```python
from build123d import *

# Parameters (mm, degrees)
SALIENTE_EXTRUIR1_DEPTH = 200


with BuildPart() as part:
    # Croquis1 → Saliente-Extruir1 (new, symmetric)
    with BuildSketch(Plane.XY):
        with BuildLine():
            Line((-10, 8.5), (-10, 2.3))
            Line((-10, 2.3), (-8.2, 2.3))
            Line((-8.2, 2.3), (-8.2, 5.5))
            Line((-8.2, 5.5), (-6.348528137, 5.5))
            Line((-6.348528137, 5.5), (-4.485786438, 3.6372583))
            ThreePointArc((-4.485786438, 3.6372583), (-4.052240935, 2.988411603), (-3.9, 2.223044738))
            Line((-3.9, 2.223044738), (-3.9, 0))
            Line((-3.9, 0), (-3.9, -2.223044738))
            ThreePointArc((-3.9, -2.223044738), (-4.052240935, -2.988411603), (-4.485786438, -3.6372583))
            Line((-4.485786438, -3.6372583), (-6.348528137, -5.5))
            Line((-6.348528137, -5.5), (-8.2, -5.5))
            Line((-8.2, -5.5), (-8.2, -2.3))
            Line((-8.2, -2.3), (-10, -2.3))
            Line((-10, -2.3), (-10, -8.5))
            ThreePointArc((-10, -8.5), (-9.560660172, -9.560660172), (-8.5, -10))
            Line((-8.5, -10), (-2.3, -10))
            Line((-2.3, -10), (-2.3, -8.2))
            Line((-2.3, -8.2), (-5.5, -8.2))
            Line((-5.5, -8.2), (-5.5, -6.348528137))
            Line((-5.5, -6.348528137), (-3.6372583, -4.485786438))
            ThreePointArc((-3.6372583, -4.485786438), (-2.988411603, -4.052240935), (-2.223044738, -3.9))
            Line((-2.223044738, -3.9), (0, -3.9))
            Line((0, -3.9), (2.223044738, -3.9))
            ThreePointArc((2.223044738, -3.9), (2.988411603, -4.052240935), (3.6372583, -4.485786438))
            Line((3.6372583, -4.485786438), (5.5, -6.348528137))
            Line((5.5, -6.348528137), (5.5, -8.2))
            Line((5.5, -8.2), (2.3, -8.2))
            Line((2.3, -8.2), (2.3, -10))
            Line((2.3, -10), (17.7, -10))
            Line((17.7, -10), (17.7, -8.2))
            Line((17.7, -8.2), (14.5, -8.2))
            Line((14.5, -8.2), (14.5, -6.348528137))
            Line((14.5, -6.348528137), (16.3627417, -4.485786438))
            ThreePointArc((16.3627417, -4.485786438), (17.011588397, -4.052240935), (17.776955262, -3.9))
            Line((17.776955262, -3.9), (20, -3.9))
            Line((20, -3.9), (22.223044738, -3.9))
            ThreePointArc((22.223044738, -3.9), (22.988411603, -4.052240935), (23.6372583, -4.485786438))
            Line((23.6372583, -4.485786438), (25.5, -6.348528137))
            Line((25.5, -6.348528137), (25.5, -8.2))
            Line((25.5, -8.2), (22.3, -8.2))
            Line((22.3, -8.2), (22.3, -10))
            Line((22.3, -10), (28.5, -10))
            ThreePointArc((28.5, -10), (29.560660172, -9.560660172), (30, -8.5))
            Line((30, -8.5), (30, -2.3))
            Line((30, -2.3), (28.2, -2.3))
            Line((28.2, -2.3), (28.2, -5.5))
            Line((28.2, -5.5), (26.348528137, -5.5))
            Line((26.348528137, -5.5), (24.485786438, -3.6372583))
            ThreePointArc((24.485786438, -3.6372583), (24.052240935, -2.988411603), (23.9, -2.223044738))
            Line((23.9, -2.223044738), (23.9, 0))
            Line((23.9, 0), (23.9, 2.223044738))
            ThreePointArc((23.9, 2.223044738), (24.052240935, 2.988411603), (24.485786438, 3.6372583))
            Line((24.485786438, 3.6372583), (26.348528137, 5.5))
            Line((26.348528137, 5.5), (28.2, 5.5))
            Line((28.2, 5.5), (28.2, 2.3))
            Line((28.2, 2.3), (30, 2.3))
            Line((30, 2.3), (30, 8.5))
            ThreePointArc((30, 8.5), (29.560660172, 9.560660172), (28.5, 10))
            Line((28.5, 10), (22.3, 10))
            Line((22.3, 10), (22.3, 8.2))
            Line((22.3, 8.2), (25.5, 8.2))
            Line((25.5, 8.2), (25.5, 6.348528137))
            Line((25.5, 6.348528137), (23.6372583, 4.485786438))
            ThreePointArc((23.6372583, 4.485786438), (22.988411603, 4.052240935), (22.223044738, 3.9))
            Line((22.223044738, 3.9), (20, 3.9))
            Line((20, 3.9), (17.776955262, 3.9))
            ThreePointArc((17.776955262, 3.9), (17.011588397, 4.052240935), (16.3627417, 4.485786438))
            Line((16.3627417, 4.485786438), (14.5, 6.348528137))
            Line((14.5, 6.348528137), (14.5, 8.2))
            Line((14.5, 8.2), (17.7, 8.2))
            Line((17.7, 8.2), (17.7, 10))
            Line((17.7, 10), (2.3, 10))
            Line((2.3, 10), (2.3, 8.2))
            Line((2.3, 8.2), (5.5, 8.2))
            Line((5.5, 8.2), (5.5, 6.348528137))
            Line((5.5, 6.348528137), (3.6372583, 4.485786438))
            ThreePointArc((3.6372583, 4.485786438), (2.988411603, 4.052240935), (2.223044738, 3.9))
            Line((2.223044738, 3.9), (0, 3.9))
            Line((0, 3.9), (-2.223044738, 3.9))
            ThreePointArc((-2.223044738, 3.9), (-2.988411603, 4.052240935), (-3.6372583, 4.485786438))
            Line((-3.6372583, 4.485786438), (-5.5, 6.348528137))
            Line((-5.5, 6.348528137), (-5.5, 8.2))
            Line((-5.5, 8.2), (-2.3, 8.2))
            Line((-2.3, 8.2), (-2.3, 10))
            Line((-2.3, 10), (-8.5, 10))
            ThreePointArc((-8.5, 10), (-9.560660172, 9.560660172), (-10, 8.5))
        make_face()
        with BuildLine():
            Line((3.9, 2.223044738), (3.9, 0))
            Line((3.9, 0), (3.9, -2.223044738))
            ThreePointArc((3.9, -2.223044738), (4.052240935, -2.988411603), (4.485786438, -3.6372583))
            Line((4.485786438, -3.6372583), (6.333883476, -5.485355339))
            ThreePointArc((6.333883476, -5.485355339), (6.604849416, -5.890884525), (6.7, -6.369238816))
            Line((6.7, -6.369238816), (6.7, -8.2))
            Line((6.7, -8.2), (13.3, -8.2))
            Line((13.3, -8.2), (13.3, -6.369238816))
            ThreePointArc((13.3, -6.369238816), (13.395150584, -5.890884525), (13.666116524, -5.485355339))
            Line((13.666116524, -5.485355339), (15.514213562, -3.6372583))
            ThreePointArc((15.514213562, -3.6372583), (15.947759065, -2.988411603), (16.1, -2.223044738))
            Line((16.1, -2.223044738), (16.1, 0))
            Line((16.1, 0), (16.1, 2.223044738))
            ThreePointArc((16.1, 2.223044738), (15.947759065, 2.988411603), (15.514213562, 3.6372583))
            Line((15.514213562, 3.6372583), (13.666116524, 5.485355339))
            ThreePointArc((13.666116524, 5.485355339), (13.395150584, 5.890884525), (13.3, 6.369238816))
            Line((13.3, 6.369238816), (13.3, 8.2))
            Line((13.3, 8.2), (6.7, 8.2))
            Line((6.7, 8.2), (6.7, 6.369238816))
            ThreePointArc((6.7, 6.369238816), (6.604849416, 5.890884525), (6.333883476, 5.485355339))
            Line((6.333883476, 5.485355339), (4.485786438, 3.6372583))
            ThreePointArc((4.485786438, 3.6372583), (4.052240935, 2.988411603), (3.9, 2.223044738))
        make_face(mode=Mode.SUBTRACT)
        with BuildLine():
            ThreePointArc((0, 2.5), (-1.767766953, 1.767766953), (-2.5, 0))
            ThreePointArc((-2.5, 0), (-1.767766953, -1.767766953), (0, -2.5))
            ThreePointArc((0, -2.5), (1.767766953, -1.767766953), (2.5, 0))
            ThreePointArc((2.5, 0), (1.767766953, 1.767766953), (0, 2.5))
        make_face(mode=Mode.SUBTRACT)
        with BuildLine():
            ThreePointArc((20, 2.5), (18.232233047, 1.767766953), (17.5, 0))
            ThreePointArc((17.5, 0), (18.232233047, -1.767766953), (20, -2.5))
            ThreePointArc((20, -2.5), (21.767766953, -1.767766953), (22.5, 0))
            ThreePointArc((22.5, 0), (21.767766953, 1.767766953), (20, 2.5))
        make_face(mode=Mode.SUBTRACT)
    extrude(amount=SALIENTE_EXTRUIR1_DEPTH, both=True)


solid = part.part
```
Part model, mm, in its own coordinate system. Coordinates: 2 decimals unless noted, no trailing zeros. Return JSON: item names as keys, results as strings. Group by question number.
Item 1: Drill centre lines: probe 1 along X at (y, z) = (-2.75, 166.5); probe 2 along X at (y, z) = (8.5, -51); probe 3 along X at (y, z) = (1, 160). Where is each one in solid material? Low to high. Write a range as from..to.
Item 2: Cut at A-A (z = 166.5). State how many separate pieces and enclosed holes the cut face has, plus the area to 3 significant figures.
Item 3: Pin check, flat tips, straight feed: pin 1 (1.5 mm diameter, centred on x = 13.5, y = -1.5, fed in from -Z); pin 2 (2 mm diameter, centred on y = -1, z = 97.5, fed in from -X); pin 3 (0.5 mm diameter, centred on y = 9.5, z = -84, fed in from -X); pin 4 (0.5 mm diameter, centred on y = 9.5, z = 40.5, fed in from +X). Stop position of each tip, or through.
Check values:
{
 "1": {"probe 1": "x = -10..-8.2, -3.97..3.97, 16.03..23.97, 28.2..30", "probe 2": "x = -10..-2.3, 2.3..17.7, 22.3..30", "probe 3": "x = -3.9..-2.29, 2.29..3.9, 16.1..17.71, 22.29..23.9"},
 "2": {"separate pieces": "1", "enclosed holes": "3", "area": "304 mm2"},
 "3": {"pin 1": "passes through", "pin 2": "stops at x = -3.9", "pin 3": "stops at x = -9.8", "pin 4": "stops at x = 29.8"}
}
